Design review of the part built by this model. Coordinates are the model's own, in mm. A direction names the side the tool comes from. Coordinates: 2 decimals unless noted, no trailing zeros. Loops run counter-clockwise (first coordinate to the right, second up) from the corner with the lowest first, then second, coordinate; pieces in that order, holes last. Notation, with made-up numbers: (-1.5, 30.5) -> (23.5, 30.5) arc R35 cw to (23.5, 64.5) -> close; hole circle Ø11 at (21.5, -5). An arc over 180 degrees is marked (long way). One line per item, written item: value. Start each with the question number.
1. Machinability: for faces 4 (the flat face through (2, 25.2, 30)), 5 (the conical face through (-1.291, 29.821, 53.114)), 6 (the flat face through (-5.6, 16, 50)), which of the approach directions +Z, -Z, +X, -X, +Y, -Y give a long, thin tool a straight path to every point of the face, cutting with its end or side? Answer none if there is none.
2. Add section D-D on x = 14.5. Write out the cut boundary in (y, z), plus the area to 3 significant figures.
3. For probe 1 along Z at (x, y) = (0, -17.3); probe 2 along Y at (x, z) = (-4, 19); probe 3 along Y at (x, z) = (-12.5, 51), list the stretches that pass through material, from the lowest coordinate up.
4. Add section B-B on z = 50. Give the number of separate pieces and of enclosed holes in the cut face, plus the area to 3 significant figures.
5. Add section C-C on x = -11.5. Write out the cut boundary in (y, z).
6. Insertion check: pin 1 (25 mm diameter, centred on x = 0, y = 0, fed in from -Z). The pin has a flat end and moves straight along its axis. Give the tip position at first contact, or say it passes through.
7. Add section A-A on y = 0. Write out the cut boundary in (x, z).
8. Draft analysis for pull direction Z (two halves, no side actions). For faces 1 (the flat face through (10, 13, 0)), 2 (the cylindrical face through (-1.245, 21.535, 53.002)), 3 (the flat face through (29, 6, 30)), state which applies: pulls with the +Z half, pulls with the -Z half, needs draft (parallel to the pull), parting line crosses it, or undercut.
```python
from build123d import *

# Parameters (mm, degrees)
SKETCH1_W           = 43
SKETCH1_H           = 43
SKETCH1_R           = 13.75
SKETCH1_H_2         = 7
BOSS_EXTRUDE1_DEPTH = 60
SKETCH3_R           = 3.25
CUT_EXTRUDE5_DEPTH  = 85.038324591
CHAMFER2_SIZE       = 2.5
CUT_EXTRUDE6_START  = -38
CUT_EXTRUDE6_DEPTH  = 15
FILLET1_R           = 10


with BuildPart() as part:
    # Sketch1 → Boss-Extrude1 (new body)
    # profile 1 of 3: a face of its own
    with BuildSketch(Plane.XY):
        with Locations((2.5, 2.5)):
            Rectangle(SKETCH1_W, SKETCH1_H)
        Circle(SKETCH1_R, mode=Mode.SUBTRACT)
    # profile 2 of 3: a face of its own
    with BuildSketch(Plane.XY):
        with Locations((2.5, 28.7)):
            Rectangle(SKETCH1_W, SKETCH1_H_2)
    # profile 3 of 3: a face of its own
    with BuildSketch(Plane.XY):
        Polygon((24, 24), (24, -19), (29, -19), (29, 32.2), (24, 32.2), (24, 25.2), align=None)
    extrude(amount=BOSS_EXTRUDE1_DEPTH)

    # Sketch3 → Cut-Extrude5 (cut, through all)
    with BuildSketch(Plane(origin=(0, 32.2, 0), x_dir=(1, 0, 0), z_dir=(0, 1, 0))):
        with Locations(Location((0, -50, 0), (0, 0, 270))):
            Circle(SKETCH3_R)
        with Locations(Location((0, -10, 0), (0, 0, 270))):
            Circle(SKETCH3_R)
    extrude(amount=-CUT_EXTRUDE5_DEPTH, mode=Mode.SUBTRACT)

    # Chamfer2
    chamfer2_edges = [part.edges().sort_by_distance(p)[0] for p in [
        (0, 32.2, 46.75),
        (0, 32.2, 6.75),
    ]]
    chamfer(chamfer2_edges, length=CHAMFER2_SIZE)

    # Sketch7 → Cut-Extrude6 (cut)
    with BuildSketch(Plane.XZ.offset(19).offset(CUT_EXTRUDE6_START)):
        Polygon((0, 43.533676985), (5.6, 46.766838493), (5.6, 53.233161507), (0, 56.466323015), (-5.6, 53.233161507), (-5.6, 46.766838493), align=None)
        Polygon((-5.6, 13.233161507), (0, 16.466323015), (5.6, 13.233161507), (5.6, 6.766838493), (0, 3.533676985), (-5.6, 6.766838493), align=None)
    extrude(amount=CUT_EXTRUDE6_DEPTH, mode=Mode.SUBTRACT)

    # Fillet1
    # the kernel refuses this fillet: 10 mm, written as the material it takes off along each edge
    with BuildSketch(Plane(origin=(-19, -19, -25), x_dir=(1, 0, 0), z_dir=(0, 0, 1)), Plane(origin=(29, 32.2, -25), x_dir=(-1, 0, 0), z_dir=(0, 0, 1)), Plane(origin=(29, -19, -25), x_dir=(0, 1, 0), z_dir=(0, 0, 1))) as fillet1_piece_1:
        with BuildLine():
            CenterArc((FILLET1_R, FILLET1_R), FILLET1_R, 180, 90)
            Line((0, FILLET1_R), (-FILLET1_R * 0.02, FILLET1_R))
            Line((-FILLET1_R * 0.02, FILLET1_R), (-FILLET1_R * 0.02, -FILLET1_R * 0.02))
            Line((-FILLET1_R * 0.02, -FILLET1_R * 0.02), (FILLET1_R, -FILLET1_R * 0.02))
            Line((FILLET1_R, -FILLET1_R * 0.02), (FILLET1_R, 0))
        make_face()
    extrude(amount=110, mode=Mode.SUBTRACT)
    with BuildSketch(Plane(origin=(-19, 32.2, -23.848480035), x_dir=(1, 0, 0), z_dir=(0, 0, 1))) as fillet1_piece_2:
        with BuildLine():
            CenterArc((9.539392014, -10), FILLET1_R, 90, 72.542396876)
            Line((0, -7), (-0.19078784, -6.94))
            ThreePointArc((-0.19078784, -6.94), (-0.2, -3.5), (-0.2, 0))
            Line((-0.2, 0), (0, 0.2))
            Line((0, 0.2), (9.539392014, 0.2))
            Line((9.539392014, 0.2), (9.539392014, 0))
        make_face()
    extrude(amount=107.696960071, mode=Mode.SUBTRACT)


solid = part.part
```
Worked answers:
1. face 4: +Z, -Z, -X
1. face 5: +Y
1. face 6: none
2. outline: (-19, 0) -> (24, 0) -> (24, 60) -> (-19, 60) -> close; (25.2, 0) -> (32.2, 0) -> (32.2, 60) -> (25.2, 60) -> close
2. area: 3,000 mm²
3. probe 1: z = 0 to 6.75, 13.25 to 46.75, 53.25 to 60
3. probe 2: y = -19 to -13.16, 13.16 to 24, 25.2 to 32.2
3. probe 3: y = -18.37 to -5.73, 5.73 to 24, 25.2 to 31.73
4. separate pieces: 3
4. enclosed holes: 0
4. area: 1,550 mm²
5. outline: (-18.68, 0) -> (-7.54, 0) -> (-7.54, 60) -> (-18.68, 60) -> close; (7.54, 0) -> (24, 0) -> (24, 60) -> (7.54, 60) -> close; (25.2, 0) -> (31.99, 0) -> (31.99, 60) -> (25.2, 60) -> close
6. pin 1: passes through
7. outline: (-19, 0) -> (-13.75, 0) -> (-13.75, 60) -> (-19, 60) -> close; (13.75, 0) -> (29, 0) -> (29, 60) -> (13.75, 60) -> close
8. face 1: pulls with the -Z half
8. face 2: undercut
8. face 3: needs draft
